Job drawing, mm, ordinate dimensions from the low corner. One solid piece. A direction names the side the tool comes from. Give positions to 0.01 mm unless a question says otherwise; leave off trailing zeros. Order: outer loops, then holes, each group sorted by start corner. A loop starts at its lowest first (then second) coordinate and runs counter-clockwise, first axis right, second up. Notation, with made-up numbers: (-8.75, 83) - (11.25, 83) arc R25 cw to (11.25, 97) - close; hole circle Ø3 at (78, 44). An arc over 180 degrees is marked (long way). One line per item, written item: value.
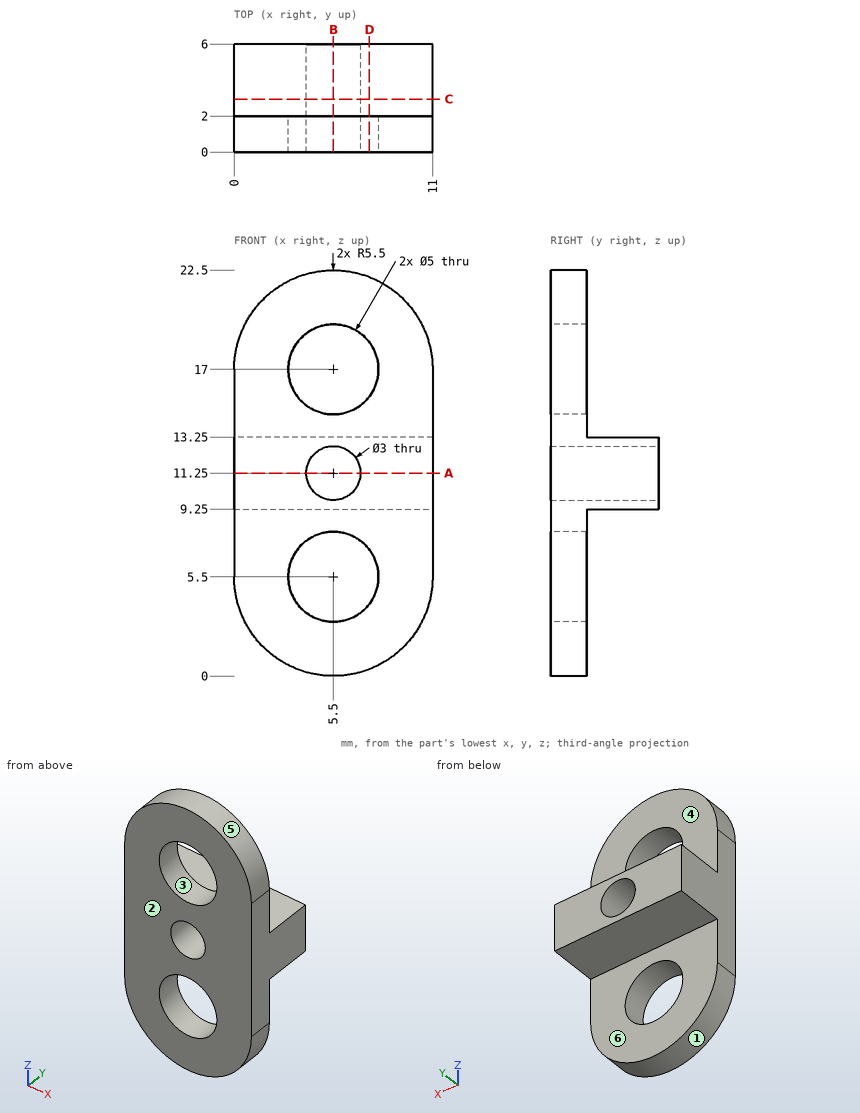
1) Slice it at A-A on z = 11.25. Write the cut outline in (x, y).
Answer:
outline: (0, 0) - (4, 0) - (4, 6) - (0, 6) - close; (7, 0) - (11, 0) - (11, 6) - (7, 6) - close
2) Two-plate mould, pull along X, no slides. Class the marked faces 1, 2 and 3: pulls with the +X half, pulls with the -X half, needs draft (parallel to the pull), parting line crosses it, or undercut.
Answer:
face 1: parting line crosses it
face 2: needs draft
face 3: undercut
3) Slice it at C-C on y = 2.95. Write the cut outline in (x, z).
Answer:
outline: (0, 9.25) - (11, 9.25) - (11, 13.25) - (0, 13.25) - close; hole circle Ø3 at (5.5, 11.25)
4) Drop flat-ended pins along their axis: P1, Ø4, axis at x = 5.5, z = 5.5, coming from the +Y side; P2, Ø2, axis at x = 6, z = 7, coming from the +Y side. Give the stop position or say it passes through.
Answer:
P1: passes through
P2: stops at y = 2
5) Wall check: line 1 along Z through (x, y) = (5.5, 0.7); line 2 along X through (y, z) = (1.5, 5.5); line 3 along X through (y, z) = (4.05, 11.25). Give the ranges that are in metal, low to high. Write a range as [from, to].
Answer:
line 1: z = [0, 3], [8, 9.75], [12.75, 14.5], [19.5, 22.5]
line 2: x = [0, 3], [8, 11]
line 3: x = [0, 4], [7, 11]
6) Slice it at B-B on x = 5.5. Write the cut outline in (y, z).
Answer:
outline: (0, 0) - (2, 0) - (2, 3) - (0, 3) - close; (0, 8) - (2, 8) - (2, 9.25) - (6, 9.25) - (6, 9.75) - (0, 9.75) - close; (0, 12.75) - (6, 12.75) - (6, 13.25) - (2, 13.25) - (2, 14.5) - (0, 14.5) - close; (0, 19.5) - (2, 19.5) - (2, 22.5) - (0, 22.5) - close
7) Slice it at D-D on x = 7.5. Write the cut outline in (y, z), then the cut area to 3 significant figures.
Answer:
outline: (0, 0.38) - (2, 0.38) - (2, 4) - (0, 4) - close; (0, 7) - (2, 7) - (2, 9.25) - (6, 9.25) - (6, 13.25) - (2, 13.25) - (2, 15.5) - (0, 15.5) - close; (0, 18.5) - (2, 18.5) - (2, 22.12) - (0, 22.12) - close
area: 47.5 mm2
8) Which spindle directions (+Z, -Z, +X, -X, +Y, -Y) get a long thin tool onto all of the face, cutting with end or side? Do the marked faces 4, 5 and 6. Say none if no direction does.
Answer:
face 4: +Z, +X, -X, +Y
face 5: +Z, +Y, -Y
face 6: -Z, +X, -X, +Y
